Read the model definition and answer for the solid it produces. Units are mm, in the model's axes. A direction names the side the tool comes from. Round coordinates to 2 decimals unless told otherwise and drop trailing zeros. Write each loop counter-clockwise with the first axis right and the second up, starting at its lowest first coordinate (ties: lowest second). Pieces come first, ordered by that corner, then holes. Notation, with made-up numbers: (-14.5, 73.25) -> (40.5, 73.25) arc R12 cw to (40.5, 82.25) -> close; hole circle Ø10 at (55.5, 83). An arc over 180 degrees is marked (long way). Return JSON: item names as keys, results as strings. Group by question number.
(1) The mould has two halves that part along Y. Classify faces 6 (the cylindrical face through (18.9, 0.5, 1.6)), 7 (the flat face through (6, -14.4, 2)), 8 (the flat face through (46.624, 19, 2)), 9 (the cylindrical face through (15.985, -20.497, 1.565)): released by +Y, released by -Y, zero draft, split by the parting line, or undercut.
(2) A cutting plane is placed at A-A on y = 0. Give the vertices of the cut face in (x, z) (3 decimals).
(3) A cutting plane is placed at C-C on x = 27.5. Give the vertices of the cut face in (y, z) (3 decimals).
(4) For faces 1 (the flat face through (11.656, -19, 2)), 2 (the flat face through (46.624, -19, 2)), 3 (the flat face through (29, -14.4, 2)), 4 (the flat face through (29, 14.4, 2)), 5 (the flat face through (11.656, 19, 2)), determine the directions among +Z, -Z, +X, -X, +Y, -Y from which every point of the face is accessible in a straight line to the end or side of a thin tool.
(5) Straight lines are drawn through the part: line 1 (X direction, y = 0, z = 2) (3 decimals); line 2 (X direction, y = -15, z = 1.75); line 3 (Y direction, x = 10, z = 0.85). For each, find the intervals that lie inside material, in ascending order.
(6) Given pin 1 (3.5 mm diameter, centred on x = 40.795, y = 0, fed in from -Z); pin 2 (1.6 mm diameter, centred on y = 17.5, z = 1, fed in from +X), each flat-ended and moving along its own axis, determine where each tip first touches the part or whether it passes through.
(7) A cutting plane is placed at B-B on z = 1.5. Give the vertices of the cut face in (x, y) (3 decimals).
```python
from build123d import *

# Parameters (mm, degrees)
SKETCH2_R           = 1.5
BOSS_EXTRUDE1_DEPTH = 3.175


with BuildPart() as part:
    # Sketch2 → Boss-Extrude1 (new body)
    with BuildSketch(Plane.XY):
        with BuildLine():
            Line((23.312, 14.4), (29.14, 14.4))
            Line((29.14, 14.4), (29.14, 0))
            Line((29.14, 0), (18.985, 0))
            ThreePointArc((18.985, 0), (17.485, 1.5), (15.985, 0))
            Line((15.985, 0), (0, 0))
            Line((0, 0), (0, 14.4))
            Line((0, 14.4), (11.656, 14.4))
            Line((11.656, 14.4), (11.656, 24.4))
            Line((11.656, 24.4), (23.312, 24.4))
            Line((23.312, 24.4), (23.312, 14.4))
        make_face()
        with Locations((17.484, 20.43125)):
            Circle(SKETCH2_R, mode=Mode.SUBTRACT)
    extrude(amount=BOSS_EXTRUDE1_DEPTH)

    # Mirror1: part across plane


with BuildPart() as part_1:
    add(part.part)
    add(part.part.mirror(Plane(origin=(0, 0, 3.175), x_dir=(0, 0, 1), z_dir=(0, 1, 0))))

    # Mirror2: part across plane


with BuildPart() as part_2:
    add(part_1.part)
    add(part_1.part.mirror(Plane(origin=(29.14, 14.4, 3.175), x_dir=(0, 0, 1), z_dir=(-1, 0, 0))))


solid = part_2.part
```
Checks:
{
 "1": {"face 6": "undercut", "face 7": "released by -Y", "face 8": "zero draft", "face 9": "undercut"},
 "2": {"outline": "(0, 0) -> (15.985, 0) -> (15.985, 3.175) -> (0, 3.175) -> close; (18.985, 0) -> (39.295, 0) -> (39.295, 3.175) -> (18.985, 3.175) -> close; (42.295, 0) -> (58.28, 0) -> (58.28, 3.175) -> (42.295, 3.175) -> close"},
 "3": {"outline": "(-14.4, 0) -> (14.4, 0) -> (14.4, 3.175) -> (-14.4, 3.175) -> close"},
 "4": {"face 1": "+Z, -Z, -X, -Y", "face 2": "+Z, -Z, +X, -Y", "face 3": "+Z, -Z, -Y", "face 4": "+Z, -Z, +Y", "face 5": "+Z, -Z, -X, +Y"},
 "5": {"line 1": "x = 0 to 15.985, 18.985 to 39.295, 42.295 to 58.28", "line 2": "x = 11.66 to 23.31, 34.97 to 46.62", "line 3": "y = -14.4 to 14.4"},
 "6": {"pin 1": "stops at z = 0", "pin 2": "stops at x = 46.62"},
 "7": {"outline": "(0, -14.4) -> (11.656, -14.4) -> (11.656, -24.4) -> (23.312, -24.4) -> (23.312, -14.4) -> (34.968, -14.4) -> (34.968, -24.4) -> (46.624, -24.4) -> (46.624, -14.4) -> (58.28, -14.4) -> (58.28, 14.4) -> (46.624, 14.4) -> (46.624, 24.4) -> (34.968, 24.4) -> (34.968, 14.4) -> (23.312, 14.4) -> (23.312, 24.4) -> (11.656, 24.4) -> (11.656, 14.4) -> (0, 14.4) -> close; hole circle Ø3 at (17.484, -20.431); hole circle Ø3 at (17.484, 20.431); hole circle Ø3 at (17.485, 0); hole circle Ø3 at (40.795, 0); hole circle Ø3 at (40.796, -20.431); hole circle Ø3 at (40.796, 20.431)"}
}
